```python
from build123d import *

# Parameters (mm, degrees)
BOSS_EXTRUDE1_DEPTH = 158.2


with BuildPart() as part:
    # Sketch3 → Boss-Extrude1 (new body)
    with BuildSketch(Plane(origin=(328.871419331, 0, 0), x_dir=(0, 0, -1), z_dir=(1, 0, 0))):
        with BuildLine():
            Line((121.186445143, 69.154189934), (121.186445143, 41.504189934))
            ThreePointArc((121.186445143, 41.504189934), (119.346896311, 32.460563946), (114.120598835, 24.854189934))
            Line((114.120598835, 24.854189934), (138.936767093, 32.389389728))
            Line((138.936767093, 32.389389728), (178.156292487, 24.854189934))
            ThreePointArc((178.156292487, 24.854189934), (172.765616446, 32.415348759), (170.862073158, 41.504189934))
            Line((170.862073158, 41.504189934), (170.862073158, 69.154189934))
            Line((170.862073158, 69.154189934), (121.186445143, 69.154189934))
        make_face()
    extrude(amount=-BOSS_EXTRUDE1_DEPTH)


solid = part.part
```
Model file for the job. Use its own axes, mm. A direction names the side the tool comes from. Give positions to 0.01 mm unless a question says otherwise; leave off trailing zeros. Order: outer loops, then holes, each group sorted by start corner. A loop starts at its lowest first (then second) coordinate and runs counter-clockwise, first axis right, second up.
1) 3-axis set-ups, long thin cutter, end or side, ignore diameter. For faces 5 (the flat face through (250.879, 28.569, -126.355)), 6 (the flat face through (251, 69.154, -146)), 7 (the flat face through (251, 55, -170.862)): which of +Z, -Z, +X, -X, +Y, -Y reach the whole face in a straight line?
2) Saw through at A-A, the plane x = 255. Write the cut outline in (y, z).
3) Saw through at C-C, the plane z = -151. Write the cut outline in (x, y).
4) Saw through at B-B, the plane y = 43. Write the cut outline in (x, z), then the cut area to 3 significant figures.
5) Pin check, flat tips, straight feed: pin 1 (1.5 mm diameter, centred on x = 249, y = 36.5, fed in from -Z); pin 2 (10 mm diameter, centred on x = 235, y = 32.5, fed in from -Z); pin 3 (12 mm diameter, centred on x = 249, z = -133.5, fed in from -Y). Stop position of each tip, or through.
6) Wall check: probe 1 along Z at (x, y) = (317, 52); probe 2 along Y at (x, z) = (294, -165); probe 3 along Z at (x, y) = (208, 37.5). Give the ranges that are in metal, low to high.
7) Mould opens along Z. For faces 1 (the flat face through (250.879, 28.675, -158.272)), 2 (the flat face through (251, 56, -121.186)), 3 (the flat face through (170.671, 47, -146)), 4 (the cylindrical face through (250.879, 32.296, -172.819)) say: +Z half, -Z half, draft (parallel to the pull), parting line (faces both ways), or undercut.
Computed:
1. face 5: +X, -X, -Y
1. face 6: +Z, -Z, +X, -X, +Y
1. face 7: -Z, +X, -X, +Y
2. outline: (24.85, -178.16) arc R22.65 cw to (41.5, -170.86) - (69.15, -170.86) - (69.15, -121.19) - (41.5, -121.19) arc R23.15 cw to (24.85, -114.12) - (32.39, -138.94) - close
3. outline: (170.67, 30.07) - (328.87, 30.07) - (328.87, 69.15) - (170.67, 69.15) - close
4. outline: (170.67, -170.86) - (328.87, -170.86) - (328.87, -121.19) - (170.67, -121.19) - close
4. area: 7,860 mm2
5. pin 1: stops at z = -171.61
5. pin 2: stops at z = -175.71
5. pin 3: stops at y = 28.92
6. probe 1: z = -170.86 to -121.19
6. probe 2: y = 27.38 to 69.15
6. probe 3: z = -171.22 to -120.84
7. face 1: undercut
7. face 2: +Z half
7. face 3: draft
7. face 4: -Z half
